Work out the finished part from the listing and answer in its coordinate system (mm). Face numbers are marked on the shaded views. A direction names the side the tool comes from. Round coordinates to 2 decimals unless told otherwise and drop trailing zeros. Order: outer loops, then holes, each group sorted by start corner. A loop starts at its lowest first (then second) coordinate and runs counter-clockwise, first axis right, second up. Notation, with made-up numbers: (16.25, -5.5) - (67.25, -5.5) arc R13 cw to (67.25, 10.5) - close; hole circle Ø6 at (88.25, 8). An arc over 180 degrees is marked (long way). Use CSV: the item, a comma, the result in double quotes.
from build123d import *

# Parameters (mm, degrees)
F0_W     = 38.1
F0_H     = 38.1
F1_DEPTH = 0.79375
F2_W     = 38.1
F2_H     = 38.1
F2_W_2   = 34.8996
F2_H_2   = 34.8996
F3_DEPTH = 5.08
F4_R     = 1.27
F5_DEPTH = 0.396875
F6_DEPTH = 4.445


with BuildPart() as f1:
    # F0 (on Top) → F1 (new body)
    with BuildSketch(Plane.XY):
        with Locations((-2.948644, 0.644133)):
            Rectangle(F0_W, F0_H)
    extrude(amount=F1_DEPTH)

    # F2 (on face) → F3 (join)
    with BuildSketch(Plane.XY.offset(0.79375)):
        with Locations((-2.948644, 0.644133)):
            Rectangle(F2_W, F2_H)
        with Locations((-2.948644, 0.644133)):
            Rectangle(F2_W_2, F2_H_2, mode=Mode.SUBTRACT)
    extrude(amount=F3_DEPTH)

    # F4 (on face) → F5 (cut)
    with BuildSketch(Plane.XY.offset(0.79375)):
        with Locations((-17.858444, -14.027401)):
            Circle(F4_R)
        with Locations((7.211356, -6.596157)):
            Circle(F4_R)
    extrude(amount=-F5_DEPTH, mode=Mode.SUBTRACT)

    # F4 (on face) → F6 (join)
    with BuildSketch(Plane.XY.offset(0.79375)):
        Polygon((-15.318444, 13.013933), (-15.318444, -16.805667), (-14.048444, -16.805667), (-14.048444, -0.956067), (-8.968444, -0.956067), (-8.968444, -5.375667), (-7.698444, -5.375667), (-7.698444, -0.956067), (-2.618444, -0.956067), (-2.618444, -10.455667), (-8.968444, -10.455667), (-8.968444, -11.725667), (-2.618444, -11.725667), (-1.348444, -11.725667), (-1.348444, -0.956067), (-1.348444, 0.313933), (-14.048444, 0.313933), (-14.048444, 11.743933), (-5.721033, 11.743933), (-5.721033, 6.663933), (-5.721033, 5.393933), (-4.451033, 5.393933), (0.894486, 5.393933), (0.894486, 6.663933), (-4.451033, 6.663933), (-4.451033, 11.743933), (9.421156, 11.743933), (9.421156, 13.013933), (-14.048444, 13.013933), align=None)
        Polygon((5.001556, -2.410417), (14.501156, -2.410417), (14.501156, -0.719784), (12.663512, -0.719784), (5.001556, -0.719784), (3.731556, -0.719784), (3.731556, -2.410417), (3.731556, -10.455667), (3.731556, -11.725667), (5.001556, -11.725667), (9.421156, -11.725667), (9.421156, -10.455667), (5.001556, -10.455667), align=None)
        Polygon((14.501156, 5.393933), (14.501156, 6.663933), (7.077073, 6.663933), (5.974486, 6.663933), (5.974486, 5.393933), (5.974486, 4.360216), (7.244486, 4.360216), (7.244486, 5.393933), align=None)
    extrude(amount=F6_DEPTH)


solid = f1.part
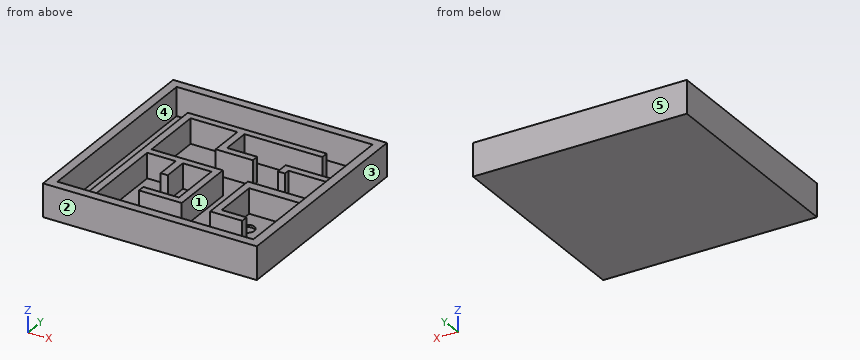
(1) Each of these flat-tipped pins is pushed along its axis until it touches: pin 1 (17.5 mm diameter, centred on x = -4, y = -1, fed in from +Z); pin 2 (1 mm diameter, centred on x = 8.5, y = -3, fed in from +Z). Where does it stop, or does it pass through?
Findings below:
pin 1,"stops at z = 5.24"
pin 2,"stops at z = 0.79"
(2) For the marked faces 4 and 5, determine the directions among +Z, -Z, +X, -X, +Y, -Y from which every point of the face is accessible in a straight line to the end or side of a thin tool.
Findings below:
face 4,"+Z"
face 5,"+Z, -Z, +X, -X, +Y"
(3) Find the intervals of material crossed by L1, parallel to Y at x = -12, z = 2.6; L2, parallel to X at y = -16.5, z = 4.8; L3, parallel to Y at x = -3.5, z = 1.4, in increasing order. Write a range as from..to.
Findings below:
L1,"y = -18.41..-16.81, -0.96..0.31, 11.74..13.01, 18.09..19.69"
L2,"x = -22..-20.4, -15.32..-14.05, 14.5..16.1"
L3,"y = -18.41..-16.81, -11.73..-10.46, -0.96..0.31, 5.39..6.66, 11.74..13.01, 18.09..19.69"
(4) Find section A-A (x = -3.5). Determine the outline of the cut face in (y, z), and give its area (3 significant figures).
Findings below:
outline,"(-18.41, 0) - (19.69, 0) - (19.69, 5.87) - (18.09, 5.87) - (18.09, 0.79) - (13.01, 0.79) - (13.01, 5.24) - (11.74, 5.24) - (11.74, 0.79) - (6.66, 0.79) - (6.66, 5.24) - (5.39, 5.24) - (5.39, 0.79) - (0.31, 0.79) - (0.31, 5.24) - (-0.96, 5.24) - (-0.96, 0.79) - (-10.46, 0.79) - (-10.46, 5.24) - (-11.73, 5.24) - (-11.73, 0.79) - (-16.81, 0.79) - (-16.81, 5.87) - (-18.41, 5.87) - close"
area,"69.1 mm²"
(5) Find section C-C (x = -10). Determine the outline of the cut face in (y, z), and give its area (3 significant figures).
Findings below:
outline,"(-18.41, 0) - (19.69, 0) - (19.69, 5.87) - (18.09, 5.87) - (18.09, 0.79) - (13.01, 0.79) - (13.01, 5.24) - (11.74, 5.24) - (11.74, 0.79) - (0.31, 0.79) - (0.31, 5.24) - (-0.96, 5.24) - (-0.96, 0.79) - (-16.81, 0.79) - (-16.81, 5.87) - (-18.41, 5.87) - close"
area,"57.8 mm²"
(6) Find section B-B (x = 12). Determine the outline of the cut face in (y, z), and give its area (3 significant figures).
Findings below:
outline,"(-18.41, 0) - (19.69, 0) - (19.69, 5.87) - (18.09, 5.87) - (18.09, 0.79) - (6.66, 0.79) - (6.66, 5.24) - (5.39, 5.24) - (5.39, 0.79) - (-0.72, 0.79) - (-0.72, 5.24) - (-2.41, 5.24) - (-2.41, 0.79) - (-16.81, 0.79) - (-16.81, 5.87) - (-18.41, 5.87) - close"
area,"59.7 mm²"
(7) The mould has two halves that part along X. Classify the marked faces 1, 2 and 3: released by +X, released by -X, zero draft, split by the parting line, or undercut.
Findings below:
face 1,"undercut"
face 2,"zero draft"
face 3,"released by +X"
